from build123d import *

# Parameters (mm, degrees)
F0_R            = 6.5
F1_DEPTH        = 11
F2_R            = 0.75
F3_DEPTH        = 6
F4_R            = 1
F5_DEPTH        = 1.5
F5_COPIES_COUNT = 3
F6_SIZE2        = 2.54
F6_SIZE         = 5.08
F7_R            = 38.1
F8_DEPTH        = 2.54


# Not quite as in the source:
# - a pattern or mirror of a feature is missing from the dataset's text; its kind, count and spacing are read off the source's solid


with BuildPart() as f1:
    # F0 (on Top) → F1 (new body)
    with BuildSketch(Plane.XY):
        Circle(F0_R)
    extrude(amount=F1_DEPTH)

    # F2 (on face) → F3 (join)
    with BuildSketch(Plane.XY.offset(11)):
        Circle(F2_R)
    extrude(amount=F3_DEPTH)

    # F4 (on face) → F5 (join)
    with BuildSketch(Plane(origin=(0, 0, 0), x_dir=(1, 0, 0), z_dir=(0, 0, -1))):
        with BuildLine():
            ThreePointArc((2, 8.6602540378), (0, 10.6602540378), (-2, 8.6602540378))
            Line((-2, 8.6602540378), (-2, 2.2360679775))
            ThreePointArc((-2, 2.2360679775), (-2.3283095216, 1.8918178485), (-2.5980762114, 1.5))
            Line((-2.5980762114, 1.5), (0, 0))
            Line((0, 0), (2.5980762114, 1.5))
            ThreePointArc((2.5980762114, 1.5), (2.3283095216, 1.8918178485), (2, 2.2360679775))
            Line((2, 2.2360679775), (2, 8.6602540378))
        make_face()
        with Locations((0, 8.6602540378)):
            Circle(F4_R, mode=Mode.SUBTRACT)
    f5 = extrude(amount=F5_DEPTH)

    # F5_copies: F5 ×3 about axis
    f5_copies_axis = Axis((0, 0, 0), (0, 0, 1))
    for i in range(1, F5_COPIES_COUNT):
        add(f5.rotate(f5_copies_axis, i * 360 / F5_COPIES_COUNT))

    # F6
    f6_edges = [f1.edges().sort_by_distance(p)[0] for p in [
        (-6.5, 0, 11),
    ]]
    f6_side = f1.faces().sort_by_distance((-6.316152, 0, 11))[0]
    chamfer(f6_edges, length=F6_SIZE, length2=F6_SIZE2, reference=f6_side)

    # F7 (on face) → F8 (join)
    with BuildSketch(Plane.XY.offset(17)):
        Circle(F7_R)
    extrude(amount=-F8_DEPTH)


solid = f1.part
Verification items for the finished model (mm, model axes). A direction names the side the tool comes from. Give positions to 0.01 mm unless a question says otherwise; leave off trailing zeros. Loops run counter-clockwise (first coordinate to the right, second up) from the corner with the lowest first, then second, coordinate; pieces in that order, holes last.
1) Depth check by flat-ended pin: pin 1 Ø8 at (x, z) = (-14, 13.5) entering from -Y; pin 2 Ø6 at (y, z) = (-7.5, 1) entering from +X; pin 3 Ø5 at (x, y) = (5, -2.5) entering from -Z. Enter the tip coordinate at first touch or a pass-through.
2) Draft check along X on faces 1 (the cylindrical face through (-5.158, -3.955, 4.171)), 2 (the cylindrical face through (8.04, 3.49, -0.74)), 3 (the flat face through (-5.68, 0.97, -0.74)). Enter one of: pulls with the +X half, pulls with the -X half, needs draft (parallel to the pull), parting line crosses it, or undercut.
3) Thickness scan on line 1 along Y through (x, z) = (-7.5, -0.65); line 2 along Z through (x, y) = (-9.5, 26.5); line 3 along X through (y, z) = (-10, 16.25). Record the ranges inside material, lowest first.
4) Set-up check for faces 4 (the flat face through (-4, -2, 0)), 5 (the flat face through (6, 4, 0)), 6 (the flat face through (-6, 4, 0)), 7 (the flat face through (1, 0, 11)): record each of +Z, -Z, +X, -X, +Y, -Y from which the full face is reachable in a straight line by a thin tool's end or side.
5) Sectioned sample at A-A, the plane x = 29. Enter the section's corners in (y, z).
6) Sectioned sample at B-B, the plane y = 24. Enter the section's corners in (x, z), then the cut area to 3 significant figures.
Answers:
1. pin 1: stops at y = -36.73
1. pin 2: stops at x = 4.69
1. pin 3: stops at z = 0
2. face 1: parting line crosses it
2. face 2: undercut
2. face 3: pulls with the -X half
3. line 1: y = 2.02 to 3.33, 5.33 to 6.33
3. line 2: z = 14.46 to 17
3. line 3: x = -36.76 to 36.76
4. face 4: -Z, -X, -Y
4. face 5: +X, +Y
4. face 6: -X, +Y
4. face 7: none
5. outline: (-24.71, 14.46) - (24.71, 14.46) - (24.71, 17) - (-24.71, 17) - close
6. outline: (-29.59, 14.46) - (29.59, 14.46) - (29.59, 17) - (-29.59, 17) - close
6. area: 150 mm2
